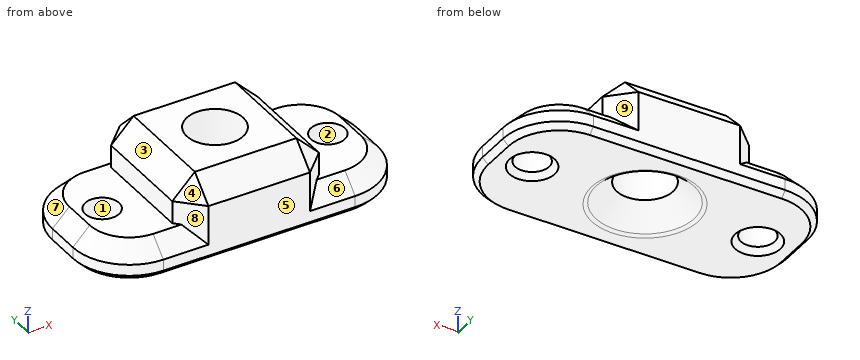
```python
from build123d import *

# Parameters (mm, degrees)
F0_W         = 13
F0_H         = 13
F0_R         = 2.5
F1_DEPTH     = 7
F0_W_2       = 7
F0_R_2       = 1.5
F2_DEPTH     = 3
F3_SIZE      = 2
F4_R         = 5
F5_SIZE      = 1.5
F6_T1_DEPTH  = 3
F6_T3_DEPTH  = 17
F6_T6_ANGLE  = 90
F6_T8_ANGLE  = 90
F6_T10_ANGLE = 90
F6_T12_ANGLE = 90


# Not quite as in the source:
# - a fillet or chamfer that OpenCascade refuses, or shapes differently, is made with other operations: its cross-section is extruded or revolved along the edge and cut away or added


with BuildPart() as f1:
    # F0 (on Top) → F1 (new body)
    with BuildSketch(Plane.XY):
        Rectangle(F0_W, F0_H)
        Circle(F0_R, mode=Mode.SUBTRACT)
    extrude(amount=F1_DEPTH)

    # F0 (on Top) → F2 (join)
    with BuildSketch(Plane.XY):
        with Locations((-10, 0)):
            Rectangle(F0_W_2, F0_H)
        with Locations((-10, 0)):
            Circle(F0_R_2, mode=Mode.SUBTRACT)
        with Locations((10, 0)):
            Rectangle(F0_W_2, F0_H)
        with Locations((10, 0)):
            Circle(F0_R_2, mode=Mode.SUBTRACT)
    extrude(amount=F2_DEPTH)

    # F3
    f3_edges = [f1.edges().sort_by_distance(p)[0] for p in [
        (-2.5, 0, 0),
        (6.5, 0, 7),
        (-6.5, 0, 7),
        (0, -6.5, 7),
        (0, 6.5, 7),
        (-6.5, -6.5, 5),
        (6.5, -6.5, 5),
        (-6.5, 6.5, 5),
        (6.5, 6.5, 5),
    ]]
    chamfer(f3_edges, length=F3_SIZE)

    # F4
    f4_edges = [f1.edges().sort_by_distance(p)[0] for p in [
        (-13.5, 6.5, 1.5),
        (-13.5, -6.5, 1.5),
        (13.5, -6.5, 1.5),
        (13.5, 6.5, 1.5),
    ]]
    fillet(f4_edges, radius=F4_R)

    # F5
    f5_edges = [f1.edges().sort_by_distance(p)[0] for p in [
        (-12.035534, -5.035534, 3),
        (12.035534, -5.035534, 3),
        (7.5, 6.5, 3),
        (12.035534, 5.035534, 3),
        (13.5, 0, 3),
        (7.5, -6.5, 3),
        (-7.5, 6.5, 3),
        (-7.5, -6.5, 3),
        (-13.5, 0, 3),
        (-12.035534, 5.035534, 3),
    ]]
    chamfer(f5_edges, length=F5_SIZE)

    # F6: chamfer of 0.5 on 11 edges, made by hand

    # F6_s2 → F6_t1 (cut)
    with BuildSketch(Plane.XZ.offset(-1.5)):
        Polygon((-13, 0), (-13.5, 0.5), (-13.5, 0), align=None)
        Polygon((13.5, 0.5), (13, 0), (13.5, 0), align=None)
    extrude(amount=F6_T1_DEPTH, mode=Mode.SUBTRACT)

    # F6_s4 → F6_t3 (cut)
    with BuildSketch(Plane.YZ.offset(-8.5)):
        Polygon((6.5, 0.5), (6, 0), (6.5, 0), align=None)
        Polygon((-6.5, 0.5), (-6, 0), (-6.5, 0), align=None)
    extrude(amount=F6_T3_DEPTH, mode=Mode.SUBTRACT)

    # F6_s5 → F6_t6 (revolve, cut)
    with BuildSketch(Plane.YZ.offset(-8.5)):
        Polygon((6, 0), (6.5, 0.5), (6.5, 0), align=None)
    revolve(axis=Axis((-8.5, 1.5, 0), (0, 0, 1)), revolution_arc=F6_T6_ANGLE, mode=Mode.SUBTRACT)

    # F6_s7 → F6_t8 (revolve, cut)
    with BuildSketch(Plane.YZ.offset(-8.5)):
        Polygon((-6, 0), (-6.5, 0.5), (-6.5, 0), align=None)
    revolve(axis=Axis((-8.5, -1.5, 0), (0, 0, -1)), revolution_arc=F6_T8_ANGLE, mode=Mode.SUBTRACT)

    # F6_s9 → F6_t10 (revolve, cut)
    with BuildSketch(Plane.YZ.offset(8.5)):
        Polygon((6.5, 0.5), (6, 0), (6.5, 0), align=None)
    revolve(axis=Axis((8.5, 1.5, 0), (0, 0, -1)), revolution_arc=F6_T10_ANGLE, mode=Mode.SUBTRACT)

    # F6_s11 → F6_t12 (revolve, cut)
    with BuildSketch(Plane.YZ.offset(8.5)):
        Polygon((-6.5, 0.5), (-6, 0), (-6.5, 0), align=None)
    revolve(axis=Axis((8.5, -1.5, 0), (0, 0, 1)), revolution_arc=F6_T12_ANGLE, mode=Mode.SUBTRACT)

    # F6_s13 → F6_t14 (revolve, cut)
    with BuildSketch(Plane.XZ):
        Polygon((4.7071067812, 0), (4.3535533906, 0.1464466094), (4.5, 0), align=None)
    revolve(axis=Axis((0, 0, 0), (0, 0, 1)), mode=Mode.SUBTRACT)

    # F6_s15 → F6_t16 (revolve, cut)
    with BuildSketch(Plane.XZ):
        Polygon((11.5, 0.5), (12, 0), (11.5, 0), align=None)
    revolve(axis=Axis((10, 0, 0), (0, 0, 1)), mode=Mode.SUBTRACT)

    # F6_s17 → F6_t18 (revolve, cut)
    with BuildSketch(Plane.XZ):
        Polygon((-8, 0), (-8.5, 0.5), (-8.5, 0), align=None)
    revolve(axis=Axis((-10, 0, 0), (0, 0, 1)), mode=Mode.SUBTRACT)


solid = f1.part
```
Can you work these out from the model? Positions are in its coordinate system, mm. Face numbers are marked on the shaded views. A direction names the side the tool comes from. Give positions to 0.01 mm unless a question says otherwise; leave off trailing zeros. Loops run counter-clockwise (first coordinate to the right, second up) from the corner with the lowest first, then second, coordinate; pieces in that order, holes last. Notation, with made-up numbers: M -31.75,57.25 L -20.75,57.25 A22 ccw -20.75,89.25 Z; hole C 72.5,4.25 d2. An arc over 180 degrees is marked long. One line per item, written item: value.
(1) Suppose I cut it at D-D on z = 2.5. List the corners of the cut face in (x, y) for me, plus the area to 3 significant figures.
Returned:
outline: M -12.5,-1.5 A4 ccw -8.5,-5.5 L -5.5,-5.5 L -4.5,-6.5 L 4.5,-6.5 L 5.5,-5.5 L 8.5,-5.5 A4 ccw 12.5,-1.5 L 12.5,1.5 A4 ccw 8.5,5.5 L 5.5,5.5 L 4.5,6.5 L -4.5,6.5 L -5.5,5.5 L -8.5,5.5 A4 ccw -12.5,1.5 Z; hole C -10,0 d3; hole C 0,0 d5; hole C 10,0 d3
area: 247 mm^2
(2) Suppose I cut it at C-C on y = 0. Count the separate pieces of the cut face and the enclosed holes in it, plus the area to 3 significant figures.
Returned:
separate pieces: 4
enclosed holes: 0
area: 69.0 mm^2
(3) Suppose I cut it at B-B on x = 7.5. List the corners of the cut face in (y, z) for me.
Returned:
outline: M -6.5,0.5 L -6,0 L 6,0 L 6.5,0.5 L 6.5,1.5 L 5,3 L -5,3 L -6.5,1.5 Z
(4) Will these pins go through, and if not, where does the flat tip stop? pin 1 (1.5 mm diameter, centred on y = -4, z = 5.5, fed in from +X); pin 2 (3.5 mm diameter, centred on x = -10, y = 0, fed in from -Z); pin 3 (5 mm diameter, centred on x = 10.5, y = -1, fed in from +Z).
Returned:
pin 1: x = 6.5
pin 2: z = 0.25
pin 3: z = 3
(5) Suppose I cut it at A-A on z = 5.75. List the corners of the cut face in (x, y) for me.
Returned:
outline: M -5.75,-4.5 L -4.5,-5.75 L 4.5,-5.75 L 5.75,-4.5 L 5.75,4.5 L 4.5,5.75 L -4.5,5.75 L -5.75,4.5 Z; hole C 0,0 d5
(6) I need wall thicknesses on line 1 (Y direction, x = -10, z = 2.1); line 2 (Y direction, x = 0, z = 5.45); line 3 (Y direction, x = 3.75, z = 5.25). Which ranges of each line are inside material? Lowest first, please.
Returned:
line 1: -5.64 to -1.5, 1.5 to 5.64
line 2: -6.05 to -2.5, 2.5 to 6.05
line 3: -6.25 to 6.25
(7) We'd pull the mould along Y, two halves only. Please class the marked faces 1, 2, 3 and 4: released by +Y, released by -Y, zero draft, split by the parting line, or undercut.
Returned:
face 1: undercut
face 2: undercut
face 3: zero draft
face 4: released by -Y
(8) Which directions (+Z, -Z, +X, -X, +Y, -Y) give clear straight access to the entire face, cutting with the end or side of a thin tool? Please do the marked faces 5, 6, 7, 8 and 9.
Returned:
face 5: +Z, -Z, +X, -X, -Y
face 6: +Z, +X, -Y
face 7: +Z, -X, +Y
face 8: +Z, -X, -Y
face 9: +Z, +X, +Y
